from build123d import *

# Parameters (mm, degrees)
SKETCH1_W               = 8
SKETCH1_H               = 8
BOSS_EXTRUDE1_DEPTH     = 3
CUT_EXTRUDE1_DEPTH      = 12.704699911
CUT_EXTRUDE1_DEPTH_BACK = 12.704699911
CUT_EXTRUDE2_DEPTH      = 11
SKETCH4_R               = 1.8
CUT_EXTRUDE3_DEPTH      = 0.8
SKETCH5_W               = 8
SKETCH5_H               = 1
BOSS_EXTRUDE2_DEPTH     = 2
FILLET1_R               = 4
CUT_EXTRUDE4_DEPTH      = 0.4


with BuildPart() as part:
    # Sketch1 → Boss-Extrude1 (new body)
    with BuildSketch(Plane(origin=(0, 0, 0), x_dir=(1, 0, 0), z_dir=(0, 1, 0))):
        with Locations((4, 4)):
            Rectangle(SKETCH1_W, SKETCH1_H)
    extrude(amount=BOSS_EXTRUDE1_DEPTH)

    # Sketch2 → Cut-Extrude1 (cut, two sides: drawn at the far end of the back side and taken through both)
    with BuildSketch(Plane.XY.offset(-CUT_EXTRUDE1_DEPTH_BACK)):
        Polygon((0, 0), (0.6, 3), (0, 3), align=None)
        Polygon((8, 0), (7.4, 3), (8, 3), align=None)
    extrude(amount=CUT_EXTRUDE1_DEPTH + CUT_EXTRUDE1_DEPTH_BACK, mode=Mode.SUBTRACT)

    # Sketch3 → Cut-Extrude2 (cut)
    with BuildSketch(Plane(origin=(0, 0, 0), x_dir=(0, 0, -1), z_dir=(1, 0, 0))):
        Polygon((0, 0), (0.6, 3), (0, 3), align=None)
        Polygon((8, 3), (7.4, 3), (8, 0), align=None)
    extrude(amount=CUT_EXTRUDE2_DEPTH, mode=Mode.SUBTRACT)

    # Sketch4 → Cut-Extrude3 (cut)
    with BuildSketch(Plane.XZ):
        with Locations(Location((4, -3.75, 0), (0, 0, 270))):
            Circle(SKETCH4_R)
    extrude(amount=-CUT_EXTRUDE3_DEPTH, mode=Mode.SUBTRACT)

    # Sketch5 → Boss-Extrude2 (add)
    with BuildSketch(Plane.XZ):
        with Locations((4, -7.5)):
            Rectangle(SKETCH5_W, SKETCH5_H)
    extrude(amount=BOSS_EXTRUDE2_DEPTH)

    # Fillet1
    # the kernel refuses this fillet: 4 mm, written as the material it takes off along each edge
    with BuildSketch(Plane(origin=(8, -2, -16.660254038), x_dir=(0, 1, 0), z_dir=(0, 0, 1)), Plane(origin=(0, -2, 1.660254038), x_dir=(0, 1, 0), z_dir=(0, 0, -1))) as fillet1_piece_1:
        with BuildLine():
            CenterArc((4, 3.464101615), FILLET1_R, 180, 60)
            Line((0, 3.464101615), (-0.08, 3.464101615))
            Line((-0.08, 3.464101615), (-0.08, 0))
            Line((-0.08, 0), (0, -0.08))
            ThreePointArc((0, -0.08), (1, -0.08), (1.96, -0.069282032))
            Line((1.96, -0.069282032), (2, 0))
        make_face()
    extrude(amount=18.320508076, mode=Mode.SUBTRACT)

    # Sketch6 → Cut-Extrude4 (cut)
    with BuildSketch(Plane(origin=(0, 3, 0), x_dir=(1, 0, 0), z_dir=(0, 1, 0))):
        with BuildLine():
            add(Edge.make_bspline(
                [(2.089654898, 3.986528763), (2.089937962, 4.035959112), (2.090493863, 4.133033938), (2.100126328, 4.27544635), (2.112822668, 4.411953966), (2.133498637, 4.542019848), (2.157821125, 4.666252751), (2.188242102, 4.784615798), (2.224888607, 4.896693893), (2.254041192, 4.968254545), (2.268340796, 5.003355686)],
                knots=[0, 0, 0, 0, 1.141009212, 2.240794809, 3.294380675, 4.305229195, 5.280013876, 6.216333343, 7.125095522, 8, 8, 8, 8], degree=3))
            add(Edge.make_bspline(
                [(2.268340796, 5.003355686), (2.291715222, 5.053256024), (2.338189152, 5.15246979), (2.424498545, 5.292666818), (2.522325153, 5.424883974), (2.630863596, 5.548428123), (2.747342854, 5.661439376), (2.872312421, 5.758160736), (3.001332505, 5.841858689), (3.093095075, 5.883953785), (3.138533104, 5.904797994)],
                knots=[0, 0, 0, 0, 1.031372299, 2.050613973, 3.077158538, 4.108712802, 5.127684358, 6.111366908, 7.06480644, 8, 8, 8, 8], degree=3))
            add(Edge.make_bspline(
                [(3.138533104, 5.904797994), (3.169376267, 5.917449171), (3.231718165, 5.943020427), (3.328604813, 5.974934694), (3.429167615, 6.000863593), (3.532679205, 6.024041008), (3.640144595, 6.040022598), (3.750695421, 6.053422612), (3.864936689, 6.060445793), (3.94221093, 6.06137636), (3.981481822, 6.061849276)],
                knots=[0, 0, 0, 0, 0.92659354, 1.872881803, 2.832850937, 3.813025581, 4.820167273, 5.851730198, 6.908245912, 8, 8, 8, 8], degree=3))
            add(Edge.make_bspline(
                [(3.981481822, 6.061849276), (4.051799393, 6.060086645), (4.189411847, 6.056637153), (4.390424999, 6.03172188), (4.580644474, 5.989650147), (4.759426374, 5.9288409), (4.928312103, 5.852828021), (5.085989518, 5.7585427), (5.232691986, 5.647005393), (5.368136158, 5.519745635), (5.490113336, 5.376985207), (5.596345325, 5.220057705), (5.685459602, 5.049698506), (5.758850354, 4.866377637), (5.815245616, 4.669496317), (5.855991141, 4.459610063), (5.880197281, 4.23656428), (5.883057671, 4.083544992), (5.884526693, 4.00495825)],
                knots=[0, 0, 0, 0, 1.064641025, 2.083517118, 3.061799897, 4.009540929, 4.938075217, 5.861300345, 6.78508344, 7.723570974, 8.670267188, 9.622657076, 10.586935816, 11.576069104, 12.607749008, 13.683335114, 14.81022093, 16, 16, 16, 16], degree=3))
            add(Edge.make_bspline(
                [(5.884526693, 4.00495825), (5.883091601, 3.926897736), (5.880297745, 3.774928499), (5.855639782, 3.553632965), (5.816583507, 3.345276789), (5.758823703, 3.150335932), (5.687623357, 2.967322864), (5.597592073, 2.798417418), (5.493584902, 2.641379175), (5.37178097, 2.500157102), (5.2386164, 2.372167), (5.092100017, 2.261933284), (4.935570416, 2.167520211), (4.767605484, 2.091287667), (4.589299985, 2.031730764), (4.400072033, 1.989335741), (4.199824576, 1.964516346), (4.062748303, 1.961054329), (3.99269977, 1.959285173)],
                knots=[0, 0, 0, 0, 1.18845052, 2.313691126, 3.386664782, 4.412527756, 5.405809582, 6.372003093, 7.321919452, 8.268293321, 9.206237639, 10.129603466, 11.054616372, 11.9847576, 12.932764752, 13.912672021, 14.933336461, 16, 16, 16, 16], degree=3))
            add(Edge.make_bspline(
                [(3.99269977, 1.959285173), (3.921851099, 1.961058411), (3.783179897, 1.964529147), (3.580796614, 1.989272994), (3.389690252, 2.031681973), (3.209996896, 2.091448367), (3.040491004, 2.166522847), (2.882737558, 2.259971154), (2.736649357, 2.370903), (2.60237212, 2.497386547), (2.480643503, 2.638193424), (2.376784009, 2.794221956), (2.286748029, 2.961477617), (2.215173347, 3.142493932), (2.157731606, 3.335408473), (2.118579893, 3.541331287), (2.09387425, 3.75969562), (2.091087056, 3.909535694), (2.089654898, 3.986528763)],
                knots=[0, 0, 0, 0, 1.080878253, 2.11558926, 3.1052859, 4.062802436, 5.000434901, 5.928596448, 6.853693179, 7.793554778, 8.738606028, 9.68692032, 10.647726704, 11.63151566, 12.651483354, 13.714466703, 14.825613081, 16, 16, 16, 16], degree=3))
        make_face()
        with BuildLine():
            add(Edge.make_bspline(
                [(2.858885668, 4.012971071), (2.85965412, 3.957640503), (2.861142212, 3.850493912), (2.876992368, 3.694973228), (2.901046254, 3.549583199), (2.936421027, 3.414488839), (2.98111032, 3.289592419), (3.035863968, 3.174789463), (3.100455695, 3.069908984), (3.176556171, 2.977165157), (3.258890919, 2.894362796), (3.347763935, 2.822717871), (3.441518937, 2.761052648), (3.541778172, 2.712368162), (3.646455066, 2.673731696), (3.756362885, 2.645084172), (3.872048117, 2.629353868), (3.950988508, 2.627098013), (3.991097206, 2.62595184)],
                knots=[0, 0, 0, 0, 1.313550922, 2.543666373, 3.708465049, 4.810029406, 5.85539231, 6.85404609, 7.825601258, 8.772642133, 9.696587791, 10.59409323, 11.479048685, 12.35559886, 13.234601248, 14.125357077, 15.047515647, 16, 16, 16, 16], degree=3))
            add(Edge.make_bspline(
                [(3.991097206, 2.62595184), (4.031211308, 2.62707479), (4.110162334, 2.629284937), (4.225705423, 2.645336869), (4.335831051, 2.6727565), (4.440092094, 2.711194976), (4.538963761, 2.760652512), (4.632359934, 2.820935331), (4.719742254, 2.892906209), (4.801987382, 2.974505658), (4.876033724, 3.06786548), (4.940075505, 3.17272786), (4.994802176, 3.288227099), (5.039496175, 3.414406406), (5.074000367, 3.551503186), (5.097072556, 3.699589977), (5.113050883, 3.858243352), (5.114532906, 3.967789388), (5.115295924, 4.02418902)],
                knots=[0, 0, 0, 0, 0.949153107, 1.868086493, 2.754172764, 3.630100905, 4.492260106, 5.365378617, 6.254840125, 7.166615376, 8.102436631, 9.067266169, 10.06813181, 11.121736829, 12.23011542, 13.408501285, 14.665770308, 16, 16, 16, 16], degree=3))
            add(Edge.make_bspline(
                [(5.115295924, 4.02418902), (5.114434086, 4.080044083), (5.112765054, 4.18821272), (5.098229512, 4.344863246), (5.07442298, 4.490602534), (5.041329269, 4.625392829), (4.997593851, 4.74925585), (4.945357013, 4.862530314), (4.882195257, 4.964624424), (4.809756461, 5.055485317), (4.729599598, 5.135460421), (4.643086506, 5.205475199), (4.549725647, 5.26373175), (4.45042821, 5.312746734), (4.344160403, 5.349110772), (4.232002157, 5.375634395), (4.113636071, 5.391967682), (4.032549387, 5.394095071), (3.991097206, 5.395182609)],
                knots=[0, 0, 0, 0, 1.332337092, 2.580197383, 3.749299508, 4.852775005, 5.886662144, 6.878700295, 7.822989687, 8.743523536, 9.644687758, 10.519443927, 11.392806431, 12.264866173, 13.155606721, 14.065961015, 15.011303331, 16, 16, 16, 16], degree=3))
            add(Edge.make_bspline(
                [(3.991097206, 5.395182609), (3.949639786, 5.394111799), (3.868542852, 5.392017134), (3.749992261, 5.375413426), (3.637480681, 5.349680139), (3.531227894, 5.311239711), (3.431065544, 5.262695426), (3.337364104, 5.202490837), (3.249385236, 5.13259488), (3.168510191, 5.05140717), (3.094897659, 4.95975062), (3.031705485, 4.856409024), (2.977820274, 4.742511001), (2.933610582, 4.617719403), (2.900837529, 4.481690937), (2.87564871, 4.335339795), (2.861503604, 4.177780175), (2.859777069, 4.069088169), (2.858885668, 4.012971071)],
                knots=[0, 0, 0, 0, 0.981996942, 1.920933313, 2.83127778, 3.712125466, 4.592427284, 5.463259035, 6.34592384, 7.249932058, 8.173122297, 9.125107726, 10.113123258, 11.154048744, 12.256187849, 13.424658091, 14.670364834, 16, 16, 16, 16], degree=3))
        make_face(mode=Mode.SUBTRACT)
    extrude(amount=-CUT_EXTRUDE4_DEPTH, mode=Mode.SUBTRACT)


solid = part.part
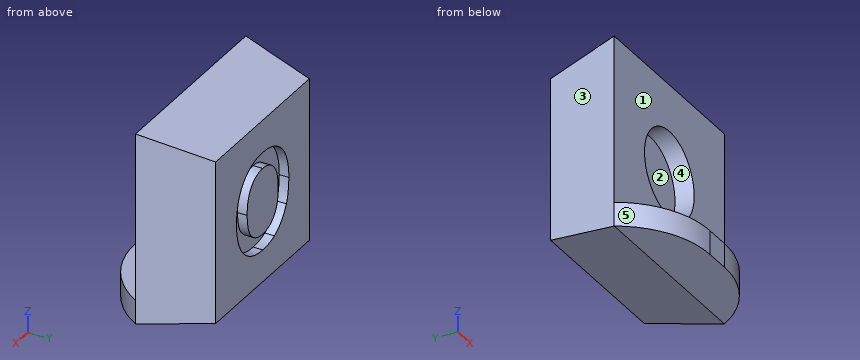
Model file for the job. Use its own axes, mm. Face numbers are marked on the shaded views. A direction names the side the tool comes from. Give positions to 0.01 mm unless a question says otherwise; leave off trailing zeros. Write each loop counter-clockwise with the first axis right and the second up, starting at its lowest first coordinate (ties: lowest second). Pieces come first, ordered by that corner, then holes. Notation, with made-up numbers: M 28.5,31.5 L 38.5,31.5 A17 ccw 38.5,55.5 Z; hole C 62,49.25 d5. An arc over 180 degrees is marked long. One line per item, written item: value. Start each with the question number.
Q1. Drop flat-ended pins along their axis: pin 1 Ø1.1 at (x, z) = (3.5, -4) entering from -Y; pin 2 Ø2 at (x, y) = (2.5, 2.5) entering from +Z. Give the stop position or say it passes through.
Q2. Saw through at D-D, the plane y = 2.2. Write the cut outline in (x, z).
Q3. 3-axis set-ups, long thin cutter, end or side, ignore diameter. For the marked faces 4 and 5: which of +Z, -Z, +X, -X, +Y, -Y reach the whole face in a straight line?
Q4. Probe probe 1 along Z at (x, y) = (1.5, -0.3); probe 2 along Y at (x, z) = (7, -4.25); probe 3 along X at (y, z) = (0.65, -3.75). List the from-to ranges inside material, lowest first. Write a range as [from, to].
Q5. Saw through at A-A, the plane y = 0.2. Write the cut outline in (x, z).
Q6. Saw through at B-B, the plane y = 1. Write the cut outline in (x, z), plus the area to 3 significant figures.
Q7. Two-plate mould, pull along X, no slides. Class the marked faces 1, 2 and 3: +X half, -X half, draft (parallel to the pull), parting line (faces both ways), or undercut.
Q8. Saw through at C-C, the plane x = 6.75. Write the cut outline in (y, z).
Output values:
1. pin 1: stops at y = 0.8
1. pin 2: stops at z = -0.3
2. outline: M 0.44,-7.56 L 7.56,-7.56 L 7.56,-0.44 L 0.44,-0.44 Z
3. face 4: -Y
3. face 5: +Z, -Z, -X, -Y
4. probe 1: z = [-8, -7]
4. probe 2: y = [0, 3]
4. probe 3: x = [0.13, 2.2], [5.8, 7.87]
5. outline: M 0.04,-7.96 L 7.96,-7.96 L 7.96,-0.04 L 0.04,-0.04 Z; hole C 4,-3.75 d3.6
6. outline: M 0.2,-7.8 L 7.8,-7.8 L 7.8,-0.2 L 0.2,-0.2 Z
6. area: 57.8 mm²
7. face 1: draft
7. face 2: undercut
7. face 3: -X half
8. outline: M -1.33,-8 L 0,-8 L 3,-7.4 L 3,-0.6 L 0,0 L 0,-7 L -1.33,-7 Z
